Verification items for the finished model (mm, model axes). Face numbers are marked on the shaded views. A direction names the side the tool comes from. Coordinates: 2 decimals unless noted, no trailing zeros. Loops run counter-clockwise (first coordinate to the right, second up) from the corner with the lowest first, then second, coordinate; pieces in that order, holes last.
Q1. Sectioned sample at C-C (x = -25). Enter the section's corners in (y, z).
Q2. Sectioned sample at D-D (z = 58). Enter the section's corners in (x, y).
Q3. Sectioned sample at A-A (x = 0). Enter the section's corners in (y, z), then the cut area to 3 significant figures.
Q4. Mould release check, pull along X, two halves, no side actions. Record for the marked faces 1, 2 and 3: +X half, -X half, draft (parallel to the pull), parting line (faces both ways), or undercut.
Q5. Access from +Z, -Z, +X, -X, +Y, -Y to the whole of each face (thin tool, end or side, straight path). Record for the marked faces 4, 5 and 6.
Q6. Material ranges on probe 1 along X at (y, z) = (87.75, 15.5); probe 2 along Y at (x, z) = (-31, -57.5); probe 3 along X at (y, z) = (87, 15), recorded low to high.
Q7. Go/stop test with flat-tipped pins: P1, Ø1, axis at x = -72.5, z = 24, coming from the +Y side; P2, Ø24, axis at x = -6.5, y = 32.5, coming from the -Z side; P3, Ø21, axis at y = 45.5, z = -2.5, coming from the +X side; P4, Ø21, axis at y = 35, z = -23, coming from the -X side. Record where each tip stops, or that it passes through.
Q8. Sectioned sample at B-B (y = 28). Enter the section's corners in (x, z).
```python
from build123d import *

# Parameters (mm, degrees)
SKETCH1_R           = 125
BOSS_EXTRUDE1_DEPTH = 10
SKETCH2_W           = 10
SKETCH2_H           = 150
BOSS_EXTRUDE2_DEPTH = 70
SKETCH3_W           = 100
SKETCH3_H           = 150
BOSS_EXTRUDE3_DEPTH = 10
SKETCH4_R           = 1.5
SKETCH4_R_2         = 12.5
CUT_EXTRUDE1_DEPTH  = 10


with BuildPart() as part:
    # Sketch1 → Boss-Extrude1 (new body)
    with BuildSketch(Plane(origin=(0, 0, 0), x_dir=(1, 0, 0), z_dir=(0, 1, 0))):
        with Locations(Location((0, 0, 0), (0, 0, 270))):
            Circle(SKETCH1_R)
    extrude(amount=BOSS_EXTRUDE1_DEPTH)

    # Sketch2 → Boss-Extrude2 (add)
    with BuildSketch(Plane(origin=(0, 10, 0), x_dir=(1, 0, 0), z_dir=(0, 1, 0))):
        with Locations((-45, 0)):
            Rectangle(SKETCH2_W, SKETCH2_H)
        with Locations((45, 0)):
            Rectangle(SKETCH2_W, SKETCH2_H)
    extrude(amount=BOSS_EXTRUDE2_DEPTH)

    # Sketch3 → Boss-Extrude3 (add)
    with BuildSketch(Plane(origin=(0, 80, 0), x_dir=(1, 0, 0), z_dir=(0, 1, 0))):
        Rectangle(SKETCH3_W, SKETCH3_H)
    extrude(amount=BOSS_EXTRUDE3_DEPTH)

    # Sketch4 → Cut-Extrude1 (cut)
    with BuildSketch(Plane(origin=(0, 90, 0), x_dir=(1, 0, 0), z_dir=(0, 1, 0))):
        with Locations(Location((-15.5, 15.5, 0), (0, 0, 270))):
            Circle(SKETCH4_R)
        with Locations(Location((15.5, 15.5, 0), (0, 0, 270))):
            Circle(SKETCH4_R)
        with Locations(Location((-15.5, -15.5, 0), (0, 0, 270))):
            Circle(SKETCH4_R)
        with Locations(Location((15.5, -15.5, 0), (0, 0, 270))):
            Circle(SKETCH4_R)
        with Locations(Location((0, 0, 0), (0, 0, 270))):
            Circle(SKETCH4_R_2)
    extrude(amount=-CUT_EXTRUDE1_DEPTH, mode=Mode.SUBTRACT)


solid = part.part
```
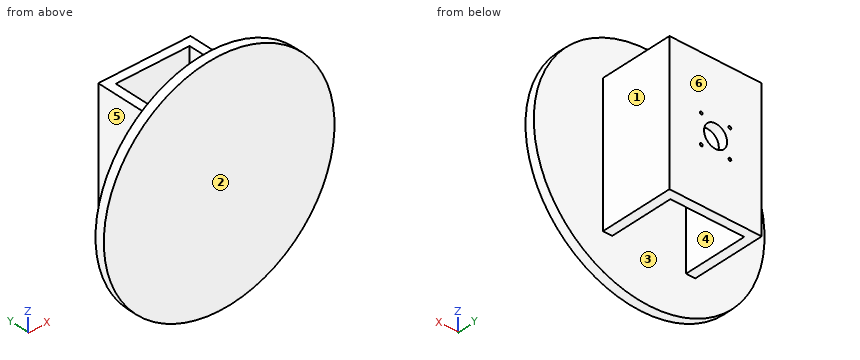
Geometry check:
1. outline: (0, -122.47) - (10, -122.47) - (10, 122.47) - (0, 122.47) - close; (80, -75) - (90, -75) - (90, 75) - (80, 75) - close
2. outline: (-110.73, 0) - (110.73, 0) - (110.73, 10) - (50, 10) - (50, 90) - (-50, 90) - (-50, 10) - (-110.73, 10) - close; hole (-40, 10) - (40, 10) - (40, 80) - (-40, 80) - close
3. outline: (0, -125) - (10, -125) - (10, 125) - (0, 125) - close; (80, -75) - (90, -75) - (90, -12.5) - (80, -12.5) - close; (80, 12.5) - (90, 12.5) - (90, 75) - (80, 75) - close
3. area: 3,750 mm2
4. face 1: +X half
4. face 2: draft
4. face 3: undercut
5. face 4: +Z, -Z
5. face 5: +Z, -Z, -X, +Y
5. face 6: +Z, -Z, +X, -X, +Y
6. probe 1: x = -50 to -17, -14 to 14, 17 to 50
6. probe 2: y = 0 to 10, 80 to 90
6. probe 3: x = -50 to -16.91, -14.09 to 14.09, 16.91 to 50
7. P1: stops at y = 10
7. P2: passes through
7. P3: stops at x = 50
7. P4: stops at x = -50
8. outline: (-50, -75) - (-40, -75) - (-40, 75) - (-50, 75) - close; (40, -75) - (50, -75) - (50, 75) - (40, 75) - close
